```python
from build123d import *

# Parameters (mm, degrees)
F0_R      = 20
F1_DEPTH  = 3
F2_R      = 5
F3_DEPTH  = 25
F4_R      = 2
F5_DEPTH  = 2
F6_R      = 8
F7_DEPTH  = 25
F8_SIZE   = 1.5
F9_R      = 28.420768
F10_DEPTH = 25


with BuildPart() as f1:
    # F0 (on Top) → F1 (new body)
    with BuildSketch(Plane.XY):
        Circle(F0_R)
    extrude(amount=F1_DEPTH)

    # F2 (on face) → F3 (cut)
    with BuildSketch(Plane.XY.offset(3)):
        Circle(F2_R)
    extrude(amount=-F3_DEPTH, mode=Mode.SUBTRACT)

    # F4 (on face) → F5 (cut)
    with BuildSketch(Plane.XY.offset(3)):
        with Locations((0, 15)):
            Circle(F4_R)
        with Locations((15, 0)):
            Circle(F4_R)
        with Locations((0, -15)):
            Circle(F4_R)
        with Locations((-15, 0)):
            Circle(F4_R)
    extrude(amount=-F5_DEPTH, mode=Mode.SUBTRACT)

    # F6 (on face) → F7 (cut)
    with BuildSketch(Plane.XY.offset(3)):
        with Locations((-10.606602, 10.606602)):
            Circle(F6_R)
        with Locations((10.606602, 10.606602)):
            Circle(F6_R)
        with Locations((10.606602, -10.606602)):
            Circle(F6_R)
        with Locations((-10.606602, -10.606602)):
            Circle(F6_R)
    extrude(amount=-F7_DEPTH, mode=Mode.SUBTRACT)

    # F8
    f8_edges = [f1.edges().sort_by_distance(p)[0] for p in [
        (-20, 0, 3),
    ]]
    chamfer(f8_edges, length=F8_SIZE)

    # F9 (on face) → F10 (cut)
    with BuildSketch(Plane.XY.offset(3)):
        with Locations((1.058917, 0)):
            Circle(F9_R)
        with BuildLine():
            ThreePointArc((-14.7, -2.984962), (-18, 0), (-14.7, 2.984962))
            ThreePointArc((-14.7, 2.984962), (-10.606602, 10.606602), (-2.984962, 14.7))
            ThreePointArc((-2.984962, 14.7), (0, 18), (2.984962, 14.7))
            ThreePointArc((2.984962, 14.7), (10.606602, 10.606602), (14.7, 2.984962))
            ThreePointArc((14.7, 2.984962), (18, 0), (14.7, -2.984962))
            ThreePointArc((14.7, -2.984962), (10.606602, -10.606602), (2.984962, -14.7))
            ThreePointArc((2.984962, -14.7), (0, -18), (-2.984962, -14.7))
            ThreePointArc((-2.984962, -14.7), (-10.606602, -10.606602), (-14.7, -2.984962))
        make_face(mode=Mode.SUBTRACT)
    extrude(amount=-F10_DEPTH, mode=Mode.SUBTRACT)


solid = f1.part
```
CAD build for the part. Positions are in the model's coordinates, mm. A direction names the side the tool comes from. Round coordinates to 2 decimals unless told otherwise and drop trailing zeros. Write each loop counter-clockwise with the first axis right and the second up, starting at its lowest first coordinate (ties: lowest second). Pieces come first, ordered by that corner, then holes. Notation, with made-up numbers: (81.5, 42.5) - (120.5, 42.5) arc R14 ccw to (120.5, 60.5) - close; hole circle Ø4 at (56, 3.5). An arc over 180 degrees is marked (long way). Return JSON: item names as keys, results as strings. Group by question number.
Item 1: 3-axis set-ups, long thin cutter, end or side, ignore diameter. For faces 1 (the face through (13.4, -1.2, 2)), 2 (the face through (-1.08, -4.88, 1.52)): which of +Z, -Z, +X, -X, +Y, -Y reach the whole face in a straight line?
Item 2: Band-saw the part on A-A on y = 0. List the corners of the cut face in (x, z), plus the area to 3 significant figures.
Item 3: Mould opens along Y. For faces 3 (the face through (18, 0, 2)), 4 (the face through (-0.1, -5.2, 0)), 5 (the face through (-4.85, -5.05, 1.52)) say: +Y half, -Y half, draft (parallel to the pull), parting line (faces both ways), or undercut.
Item 4: Probe probe 1 along Y at (x, z) = (0, 2.1); probe 2 along Y at (x, z) = (-15, 2.1); probe 3 along Y at (x, z) = (0, 0.8). List the from-to ranges inside material, lowest first.
Item 5: Band-saw the part on D-D on y = 13.5. List the corners of the cut face in (x, z), plus the area to 3 significant figures.
Item 6: Band-saw the part on C-C on z = 2.1. List the corners of the cut face in (x, y), plus the area to 3 significant figures.
Item 7: Flat gauge pins, fed straight in: pin 1 Ø1.2 at (x, y) = (0.5, -14.5) entering from +Z; pin 2 Ø1 at (x, z) = (-5.5, 0.5) entering from -Y; pin 3 Ø1 at (y, z) = (-2.5, 0.5) entering from -X. Where does each tip first touch, or does it go through?
Resolved:
{
 "1": {"face 1": "+Z", "face 2": "+Z, -Z"},
 "2": {"outline": "(-18, 0) - (-5, 0) - (-5, 3) - (-13, 3) - (-13, 1) - (-17, 1) - (-17, 3) - (-18, 3) - close; (5, 0) - (18, 0) - (18, 3) - (17, 3) - (17, 1) - (13, 1) - (13, 3) - (5, 3) - close", "area": "62.0 mm²"},
 "3": {"face 3": "parting line", "face 4": "draft", "face 5": "undercut"},
 "4": {"probe 1": "y = -18 to -17, -13 to -5, 5 to 13, 17 to 18", "probe 2": "y = -3 to -2, 2 to 3", "probe 3": "y = -18 to -5, 5 to 18"},
 "5": {"outline": "(-3.15, 0) - (3.15, 0) - (3.15, 3) - (1.32, 3) - (1.32, 1) - (-1.32, 1) - (-1.32, 3) - (-3.15, 3) - close", "area": "13.6 mm²"},
 "6": {"outline": "(-14.7, -2.98) arc R15 ccw to (-14.55, -3.65) arc R8 cw to (-3.65, -14.55) arc R15 ccw to (-2.98, -14.7) arc R3 ccw (long way) to (2.98, -14.7) arc R15 ccw to (3.65, -14.55) arc R8 cw to (14.55, -3.65) arc R15 ccw to (14.7, -2.98) arc R3 ccw (long way) to (14.7, 2.98) arc R15 ccw to (14.55, 3.65) arc R8 cw to (3.65, 14.55) arc R15 ccw to (2.98, 14.7) arc R3 ccw (long way) to (-2.98, 14.7) arc R15 ccw to (-3.65, 14.55) arc R8 cw to (-14.55, 3.65) arc R15 ccw to (-14.7, 2.98) arc R3 ccw (long way) to start; hole circle Ø4 at (-15, 0); hole circle Ø10 at (0, 0); hole circle Ø4 at (0, -15); hole circle Ø4 at (0, 15); hole circle Ø4 at (15, 0)", "area": "281 mm²"},
 "7": {"pin 1": "stops at z = 1", "pin 2": "stops at y = -4.9", "pin 3": "stops at x = -17.24"}
}
